Work out the finished part from the listing and answer in its coordinate system (mm). Face numbers are marked on the shaded views. A direction names the side the tool comes from. Round coordinates to 2 decimals unless told otherwise and drop trailing zeros. Write each loop counter-clockwise with the first axis right and the second up, starting at its lowest first coordinate (ties: lowest second). Pieces come first, ordered by that corner, then holes. Notation, with made-up numbers: M -5,51 L 27,51 A24 ccw 27,77 Z; hole C 11.25,83.5 d5. An arc over 180 degrees is marked long. One line per item, written item: value. Start each with the question number.
Q1. Find section D-D (z = -14). Write down the section's boundary in (x, y).
Q2. Given pin 1 Ø16 at (x, z) = (10.5, -9.5) entering from -Y; pin 2 Ø6 at (y, z) = (3.5, -40.5) entering from +X; pin 3 Ø6.5 at (x, y) = (9, 13.5) entering from -Z, each flat-ended and moving along its own axis, determine where each tip first touches the part or whether it passes through.
Q3. Find section B-B (z = -8). Write down the section's boundary in (x, y), and give its area (3 significant figures).
Q4. Consider probe 1 along Z at (x, y) = (9.5, 11.25); probe 2 along X at (y, z) = (4, -28); probe 3 along X at (y, z) = (11, -16.5). Determine where each line is inside the solid, lowest interval first.
Q5. A tool of negligible diameter and unlimited length cuts with its end or side. For the marked faces 1, 2, 3, 4 and 5, from which of +Z, -Z, +X, -X, +Y, -Y can it reach the whole face along a straight path? Write none if from no direction.
Q6. Find section C-C (y = 11.5). Write down the section's boundary in (x, z).
Q7. The mould has two halves that part along Z. Classify the marked faces 6, 7, 8 and 9: released by +Z, released by -Z, zero draft, split by the parting line, or undercut.
Q8. Find section A-A (x = 16). Write down the section's boundary in (y, z).
Autodesk Inventor part; units mm, degrees
ref_plane "YZ Plane" through (0, 0, 0) normal (1, 0, 0) x (0, 1, 0)
ref_plane "XZ Plane" through (0, 0, 0) normal (0, 1, 0) x (-1, 0, 0)
ref_plane "XY Plane" through (0, 0, 0) normal (0, 0, 1) x (1, 0, 0)
sketch "Sketch1" plane through (0, 0, 0) normal (0, 1, 0) x (-1, 0, 0)
  line L0 (0, 0) -> (20, 0)
  line L1 (20, 0) -> (20, -60)
  line L2 (20, -60) -> (0, -60)
  line L3 (0, -60) -> (0, 0)
  dimension "d0" = 20
  dimension "d1" = 60
extrude "Extrusion1" add sketch "Sketch1" along normal blind 17
sketch "Sketch2" plane through (0, 0, 0) normal (1, 0, 0) x (0, 0, -1)
  line L0 (60, 17) -> (0, 17)
  line L1 (0, 17) -> (10, 17)
  line L2 (10, 17) -> (10, 9)
  line L3 (10, 9) -> (0, 9)
  line L4 (0, 9) -> (0, 17)
  line L5 (10, 17) -> (20, 17)
  line L6 (20, 17) -> (30, 17)
  line L7 (30, 17) -> (30, 9)
  line L8 (30, 9) -> (20, 9)
  line L9 (20, 9) -> (20, 17)
  line L10 (10, 9) -> (20, 9)
  point P0 (0, 0)
  dimension "d4" = 10
  dimension "d5" = 8
  dimension "d6" = 10
  dimension "d7" = 10
  dimension "d8" = 8
extrude "Extrusion2" add sketch "Sketch2" along normal blind 20 contours L7 L8 L9 L0 | L2 L3 L4 L0
sketch "Sketch3" plane through (0, 17, 0) normal (0, 1, 0) x (1, 0, 0)
  point P0 (0, 0)
extrude "Extrusion3" add sketch "Sketch2" along normal blind 7 contours L9 L10 L2 L0
properties part number "millenium"
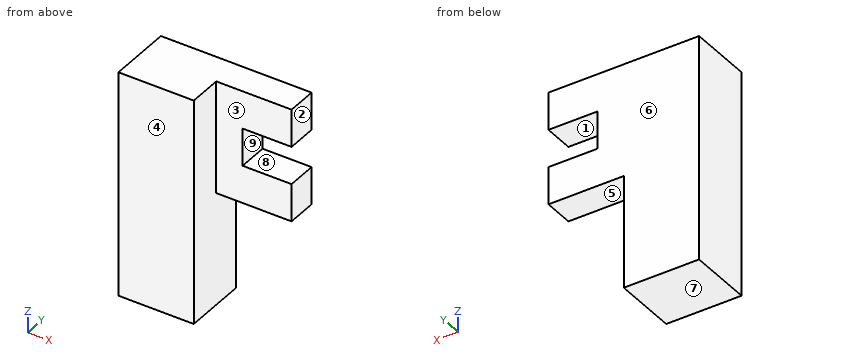
The answers:
1. outline: M -20,0 L 0,0 L 0,9 L 7,9 L 7,17 L -20,17 Z
2. pin 1: y = 9
2. pin 2: x = 0
2. pin 3: z = -30
3. outline: M -20,0 L 0,0 L 0,9 L 20,9 L 20,17 L -20,17 Z
3. area: 500 mm2
4. probe 1: -30 to -20, -10 to 0
4. probe 2: -20 to 0
4. probe 3: -20 to 7
5. face 1: +X, +Y, -Y
5. face 2: +Z, -Z, +X, +Y, -Y
5. face 3: +Z, -Z, +X, -Y
5. face 4: +Z, -Z, +X, -X, -Y
5. face 5: -Z, +X, +Y, -Y
6. outline: M -20,-60 L 0,-60 L 0,-30 L 20,-30 L 20,-20 L 7,-20 L 7,-10 L 20,-10 L 20,0 L -20,0 Z
7. face 6: zero draft
7. face 7: released by -Z
7. face 8: undercut
7. face 9: undercut
8. outline: M 9,-30 L 17,-30 L 17,-20 L 9,-20 Z; M 9,-10 L 17,-10 L 17,0 L 9,0 Z
